Design review of the part built by this model. Coordinates are the model's own, in mm. A direction names the side the tool comes from. Coordinates: 2 decimals unless noted, no trailing zeros. Order: outer loops, then holes, each group sorted by start corner. A loop starts at its lowest first (then second) coordinate and runs counter-clockwise, first axis right, second up. Notation, with made-up numbers: (-35, 8) - (9, 8) arc R10 ccw to (9, 22) - close; hole circle Ø8 at (41.25, 20). An arc over 180 degrees is marked (long way). Write item = value, one per line. Start each with the question number.
```python
from build123d import *

# Parameters (mm, degrees)
F1_DEPTH = 63.5
F3_DEPTH = 12.7
F5_DEPTH = 31.75


# Not quite as in the source:
# - a pattern or mirror of a feature is missing from the dataset's text; its kind, count and spacing are read off the source's solid


with BuildPart() as f1:
    # F0 (on Top) → F1 (new body)
    with BuildSketch(Plane.XY):
        Polygon((0, 9.525), (0, 0), (9.525, 0), align=None)
    extrude(amount=F1_DEPTH)

    # F2 (on face) → F3 (join)
    with BuildSketch(Plane.XY.offset(63.5)):
        Polygon((12.7, -3.175), (4.7625, 4.7625), (-3.175, 12.7), (-3.175, -3.175), align=None)
    extrude(amount=-F3_DEPTH)

    # F4 (on face) → F5 (join)
    with BuildSketch(Plane.XZ):
        Polygon((0, 50.8), (0, 0), (3.175, 0), (3.175, 63.5), (-3.175, 63.5), (-3.175, 50.8), align=None)
    f5 = extrude(amount=-F5_DEPTH)

    # F5_copies: F5 across plane
    add(f5.mirror(Plane(origin=(0, 0, 0), x_dir=(-0.7071067812, -0.7071067812, 0), z_dir=(0.7071067812, -0.7071067812, 0))))


solid = f1.part
```
Item 1: For P1, Ø1.5, axis at y = 12.5, z = 24, coming from the +X side (3 decimals); P2, Ø5, axis at x = 26, z = 16.5, coming from the -Y side; P3, Ø5, axis at x = 16.5, z = 8, coming from the +Y side (3 decimals), all flat-tipped, find the tip position at first contact; note any pin that passes through.
Item 2: Add section A-A on z = 40.5. Give the boundary of the cut face in (x, y) (3 decimals).
Item 3: For line 1 (Y direction, x = 29.5, z = 53) (3 decimals); line 2 (Y direction, x = 8.5, z = 35) (3 decimals), list the stretches that pass through material, from the lowest coordinate up.
Item 4: Add section B-B on y = 14. Give the boundary of the cut face in (x, z) (3 decimals).
Item 5: For faces 1 (the flat face through (19, 3.175, 31)), 2 (the flat face through (16, 0, 25)), 3 (the flat face through (1, 31.75, 39)), 4 (the flat face through (0, 16, 26)), list the 3-axis set-ups (+Z, -Z, +X, -X, +Y, -Y) from which the entire face can be reached by the end or side of a thin tool; tool diameter is ignored.
Item 6: Add section D-D on z = 58. Give the boundary of the cut face in (x, y) (3 decimals).
Worked out:
q1.P1 = 3.175
q1.P2 = 0
q1.P3 = 3.175
q2.outline = (0, 0) - (31.75, 0) - (31.75, 3.175) - (6.35, 3.175) - (3.175, 6.35) - (3.175, 31.75) - (0, 31.75) - close
q3.line_1 = -3.175 to 3.175
q3.line_2 = 0 to 3.175
q4.outline = (-3.175, 50.8) - (0, 50.8) - (0, 0) - (3.175, 0) - (3.175, 63.5) - (-3.175, 63.5) - close
q5.face_1 = +Z, -Z, +X, +Y
q5.face_2 = -Z, +X, -X, -Y
q5.face_3 = +Z, -Z, +X, -X, +Y
q5.face_4 = -Z, -X, +Y, -Y
q6.outline = (-3.175, -3.175) - (31.75, -3.175) - (31.75, 3.175) - (6.35, 3.175) - (3.175, 6.35) - (3.175, 31.75) - (-3.175, 31.75) - close
